```python
from build123d import *

# Parameters (mm, degrees)
SKETCH1_W           = 50.8
SKETCH1_H           = 33.02
BOSS_EXTRUDE1_DEPTH = 2.54
SKETCH2_R           = 3.175
SKETCH2_R_2         = 1.524
BOSS_EXTRUDE3_DEPTH = 2.54
SKETCH3_W           = 22.225
SKETCH3_H           = 2.54
SKETCH3_W_2         = 6.35
SKETCH3_W_3         = 2.54
SKETCH3_H_2         = 6.35
SKETCH3_H_3         = 17.145
SKETCH3_H_4         = 9.525
BOSS_EXTRUDE4_DEPTH = 11.43
SKETCH5_W           = 2.54
SKETCH5_H           = 9.525
CUT_EXTRUDE2_DEPTH  = 11.43
SKETCH6_R           = 1.524
BOSS_EXTRUDE7_DEPTH = 8.89


with BuildPart() as part:
    # Sketch1 → Boss-Extrude1 (new body)
    with BuildSketch(Plane(origin=(0, 0, 0), x_dir=(0, 0, -1), z_dir=(1, 0, 0))):
        with Locations((25.4, 16.51)):
            Rectangle(SKETCH1_W, SKETCH1_H)
    extrude(amount=BOSS_EXTRUDE1_DEPTH)

    # Sketch2 → Boss-Extrude3 (add)
    # profile 1 of 6: a face of its own
    with BuildSketch(Plane(origin=(2.54, 0, 0), x_dir=(0, 0, -1), z_dir=(1, 0, 0))):
        with BuildLine():
            Line((-6.35, 9.525), (0, 9.525))
            Line((0, 9.525), (0, 15.875))
            Line((0, 15.875), (-6.35, 15.875))
            ThreePointArc((-6.35, 15.875), (-4.10493597, 14.94506403), (-3.175, 12.7))
            ThreePointArc((-3.175, 12.7), (-4.10493597, 10.45493597), (-6.35, 9.525))
        make_face()
    # profile 2 of 6: a face of its own
    with BuildSketch(Plane(origin=(2.54, 0, 0), x_dir=(0, 0, -1), z_dir=(1, 0, 0))):
        with Locations((-6.35, 12.7)):
            Circle(SKETCH2_R)
        with Locations((-6.35, 12.7)):
            Circle(SKETCH2_R_2, mode=Mode.SUBTRACT)
    # profile 3 of 6: a face of its own
    with BuildSketch(Plane(origin=(2.54, 0, 0), x_dir=(0, 0, -1), z_dir=(1, 0, 0))):
        with BuildLine():
            Line((28.575, -6.35), (28.575, 0))
            Line((28.575, 0), (22.225, 0))
            Line((22.225, 0), (22.225, -6.35))
            ThreePointArc((22.225, -6.35), (25.4, -3.175), (28.575, -6.35))
        make_face()
    # profile 4 of 6: a face of its own
    with BuildSketch(Plane(origin=(2.54, 0, 0), x_dir=(0, 0, -1), z_dir=(1, 0, 0))):
        with Locations((25.4, -6.35)):
            Circle(SKETCH2_R)
        with Locations((25.4, -6.35)):
            Circle(SKETCH2_R_2, mode=Mode.SUBTRACT)
    # profile 5 of 6: a face of its own
    with BuildSketch(Plane(origin=(2.54, 0, 0), x_dir=(0, 0, -1), z_dir=(1, 0, 0))):
        with BuildLine():
            Line((50.8, 9.525), (57.15, 9.525))
            ThreePointArc((57.15, 9.525), (53.975, 12.7), (57.15, 15.875))
            Line((57.15, 15.875), (50.8, 15.875))
            Line((50.8, 15.875), (50.8, 9.525))
        make_face()
    # profile 6 of 6: a face of its own
    with BuildSketch(Plane(origin=(2.54, 0, 0), x_dir=(0, 0, -1), z_dir=(1, 0, 0))):
        with Locations((57.15, 12.7)):
            Circle(SKETCH2_R)
        with Locations((57.15, 12.7)):
            Circle(SKETCH2_R_2, mode=Mode.SUBTRACT)
    extrude(amount=-BOSS_EXTRUDE3_DEPTH)

    # Sketch3 → Boss-Extrude4 (add)
    with BuildSketch(Plane(origin=(2.54, 0, 0), x_dir=(0, 0, -1), z_dir=(1, 0, 0))):
        with Locations((39.6875, -1.27)):
            Rectangle(SKETCH3_W, SKETCH3_H)
        Polygon((22.225, 0), (0, 0), (-2.54, 0), (-2.54, -2.54), (22.225, -2.54), align=None)
        with Locations((25.4, -1.27)):
            Rectangle(SKETCH3_W_2, SKETCH3_H)
        Polygon((53.34, 9.525), (50.8, 9.525), (50.8, 0), (50.8, -2.54), (53.34, -2.54), align=None)
        with Locations((52.07, 12.7)):
            Rectangle(SKETCH3_W_3, SKETCH3_H_2)
        with Locations((52.07, 24.4475)):
            Rectangle(SKETCH3_W_3, SKETCH3_H_3)
        Polygon((50.8, 33.02), (53.34, 33.02), (53.34, 35.56), (-2.54, 35.56), (-2.54, 33.02), (0, 33.02), align=None)
        with Locations((-1.27, 24.4475)):
            Rectangle(SKETCH3_W_3, SKETCH3_H_3)
        with Locations((-1.27, 12.7)):
            Rectangle(SKETCH3_W_3, SKETCH3_H_2)
        with Locations((-1.27, 4.7625)):
            Rectangle(SKETCH3_W_3, SKETCH3_H_4)
    extrude(amount=-BOSS_EXTRUDE4_DEPTH)

    # Sketch5 → Cut-Extrude2 (cut)
    with BuildSketch(Plane.ZY.offset(8.89)):
        with Locations((-52.07, 4.7625)):
            Rectangle(SKETCH5_W, SKETCH5_H)
    extrude(amount=-CUT_EXTRUDE2_DEPTH, mode=Mode.SUBTRACT)

    # Sketch6 → Boss-Extrude7 (add)
    # profile 1 of 3: a face of its own
    with BuildSketch(Plane.ZY):
        with BuildLine():
            Line((2.54, 15.875), (2.54, 9.525))
            Line((2.54, 9.525), (6.35, 9.525))
            ThreePointArc((6.35, 9.525), (9.525, 12.7), (6.35, 15.875))
            Line((6.35, 15.875), (2.54, 15.875))
        make_face()
        with Locations(Location((6.35, 12.7, 0), (0, 0, 180))):
            Circle(SKETCH6_R, mode=Mode.SUBTRACT)
    # profile 2 of 3: a face of its own
    with BuildSketch(Plane.ZY):
        with BuildLine():
            Line((-22.225, -2.54), (-28.575, -2.54))
            Line((-28.575, -2.54), (-28.575, -6.35))
            ThreePointArc((-28.575, -6.35), (-25.4, -9.525), (-22.225, -6.35))
            Line((-22.225, -6.35), (-22.225, -2.54))
        make_face()
        with Locations(Location((-25.4, -6.35, 0), (0, 0, 180))):
            Circle(SKETCH6_R, mode=Mode.SUBTRACT)
    # profile 3 of 3: a face of its own
    with BuildSketch(Plane.ZY):
        with BuildLine():
            Line((-53.34, 15.875), (-53.34, 9.525))
            Line((-53.34, 9.525), (-57.15, 9.525))
            ThreePointArc((-57.15, 9.525), (-60.325, 12.7), (-57.15, 15.875))
            Line((-57.15, 15.875), (-53.34, 15.875))
        make_face()
        with Locations(Location((-57.15, 12.7, 0), (0, 0, 180))):
            Circle(SKETCH6_R, mode=Mode.SUBTRACT)
    extrude(amount=BOSS_EXTRUDE7_DEPTH)


solid = part.part
```
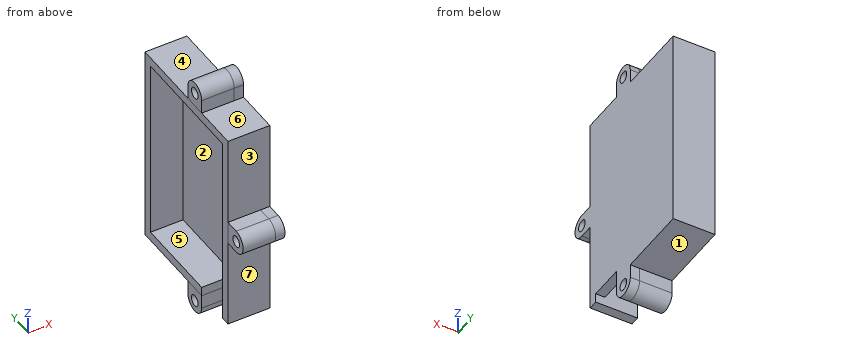
The model under review builds one solid part; all positions refer to its coordinate system, in mm. Face numbers are marked on the shaded views. A direction names the side the tool comes from. Give positions to 0.01 mm unless a question says otherwise; leave off trailing zeros. Write each loop counter-clockwise with the first axis right and the second up, starting at its lowest first coordinate (ties: lowest second). Pieces come first, ordered by that corner, then holes. Notation, with made-up numbers: (11, 59.5) - (27, 59.5) arc R8 cw to (27, 72.5) - close; hole circle Ø10 at (-6.75, 55.25). An arc over 180 degrees is marked (long way). Answer in a Markdown table with one row per item. Add a question column.
1. We need section A-A on z = -25.4. Write out the cut boundary in (x, y) (3 decimals).
2. Tool access review of the marked faces 4, 5, 6 and 7: name each direction out of +Z, -Z, +X, -X, +Y, -Y from which nothing blocks a thin tool from reaching the whole face with its end or side.
3. We need section C-C on x = -3.5. Write out the cut boundary in (y, z) (3 decimals), then the cut area to 3 significant figures.
4. Draft analysis for pull direction Z (two halves, no side actions). For the marked faces 1, 2 and 3, state which applies: +Z half, -Z half, draft (parallel to the pull), parting line (faces both ways), or undercut.
5. Insertion check: P1, Ø2.5, axis at y = 12.7, z = -57.15, coming from the +X side; P2, Ø1.3, axis at x = 1.5, z = 5, coming from the -Y side (3 decimals); P3, Ø3, axis at x = -5.5, z = -54.5, coming from the -Y side; P4, Ø6, axis at x = -1, y = 30, coming from the +Z side. Each pin has a flat end and moves straight along its axis. Give the tip position at first contact, or say it passes through.
6. We need section D-D on z = -47. Write out the cut boundary in (x, y).
7. We need section B-B on y = 12.7. Write out the cut boundary in (x, z) (3 decimals), then the cut area to 3 significant figures.
8. Wall thickness on line 1 along Z through (x, y) = (-1.75, 12.7) (3 decimals); line 2 along Y through (x, z) = (-4.25, -25.4) (3 decimals); line 3 along Y through (x, z) = (-4.5, -44): over which ranges is each line inside the solid? List them lowest first. Write a range as [from, to].
Ans:
| question | item | result |
|---|---|---|
| 1 | outline | (-8.89, -9.525) - (2.54, -9.525) - (2.54, -7.874) - (-8.89, -7.874) - close; (-8.89, -4.826) - (2.54, -4.826) - (2.54, 35.56) - (-8.89, 35.56) - (-8.89, 33.02) - (0, 33.02) - (0, 0) - (-8.89, 0) - close |
| 2 | face 4 | +Z, +X, -X, +Y |
| 2 | face 5 | -X |
| 2 | face 6 | +Z, +X, -X, -Y |
| 2 | face 7 | -Z, +X, -X, -Y |
| 3 | outline | (-6.35, -28.575) - (-2.54, -28.575) - (-2.54, -53.34) - (0, -53.34) - (0, 0) - (33.02, 0) - (33.02, -50.8) - (9.525, -50.8) - (9.525, -57.15) arc R3.175 ccw to (15.875, -57.15) - (15.875, -53.34) - (35.56, -53.34) - (35.56, 2.54) - (15.875, 2.54) - (15.875, 6.35) arc R3.175 ccw to (9.525, 6.35) - (9.525, 2.54) - (-2.54, 2.54) - (-2.54, -22.225) - (-6.35, -22.225) arc R3.175 ccw to start; hole circle Ø3.048 at (-6.35, -25.4); hole circle Ø3.048 at (12.7, -57.15); hole circle Ø3.048 at (12.7, 6.35) |
| 3 | area | 526 mm^2 |
| 4 | face 1 | -Z half |
| 4 | face 2 | undercut |
| 4 | face 3 | draft |
| 5 | P1 | passes through |
| 5 | P2 | stops at y = 9.525 |
| 5 | P3 | stops at y = -2.54 |
| 5 | P4 | stops at z = 2.54 |
| 6 | outline | (-8.89, -2.54) - (2.54, -2.54) - (2.54, 35.56) - (-8.89, 35.56) - (-8.89, 33.02) - (0, 33.02) - (0, 0) - (-8.89, 0) - close |
| 7 | outline | (-8.89, -60.325) - (2.54, -60.325) - (2.54, -58.674) - (-8.89, -58.674) - close; (-8.89, -55.626) - (2.54, -55.626) - (2.54, 4.826) - (-8.89, 4.826) - (-8.89, 0) - (0, 0) - (0, -50.8) - (-8.89, -50.8) - close; (-8.89, 7.874) - (2.54, 7.874) - (2.54, 9.525) - (-8.89, 9.525) - close |
| 7 | area | 277 mm^2 |
| 8 | line 1 | z = [-60.325, -58.674], [-55.626, -50.8], [0, 4.826], [7.874, 9.525] |
| 8 | line 2 | y = [-9.525, -7.874], [-4.826, 0], [33.02, 35.56] |
| 8 | line 3 | y = [-2.54, 0], [33.02, 35.56] |
